Here's how the part is built. I have some questions about the finished solid (model axes, mm). A direction names the side the tool comes from. Round coordinates to 2 decimals unless told otherwise and drop trailing zeros. Order: outer loops, then holes, each group sorted by start corner. A loop starts at its lowest first (then second) coordinate and runs counter-clockwise, first axis right, second up. Notation, with made-up numbers: M 31,80.5 L 58,80.5 A18 cw 58,115.5 Z; hole C 36,-5.75 d4. An arc over 180 degrees is marked long. Write item = value, one per line. Start each with the question number.
Item 1: I want a section at C-C, the plane z = 15.5. List the corners of the cut face in (x, y) for me, plus the area to 3 significant figures.
Item 2: I want a section at D-D, the plane x = 0. List the corners of the cut face in (y, z) for me, plus the area to 3 significant figures.
Item 3: I want a section at A-A, the plane y = 0. State how many separate pieces and enclosed holes the cut face has, plus the area to 3 significant figures.
Item 4: For faces 1 (the face through (0, 5, 48)), 2 (the face through (-19, 0, 29)), 3 (the face through (-17.247, 0.121, 59.479)), which set-ups out of +Z, -Z, +X, -X, +Y, -Y let a thin tool reach every point of the face, with its end or its side?
Item 5: I'm going to push flat-ended pins straight in: P1, Ø6, axis at y = -1, z = 45.5, coming from the -X side; P2, Ø3.5, axis at x = 14.5, y = 0, coming from the +Z side. Where does each tip first touch, or does it pass through?
Item 6: We'd pull the mould along Y, two halves only. Please class faces 4 (the face through (2, -10, 23)), 5 (the face through (-17, -2, 20)), 6 (the face through (20, -2, 48)): pulls with the +Y half, pulls with the -Y half, needs draft (parallel to the pull), parting line crosses it, or undercut.
Item 7: I want a section at B-B, the plane x = -14.5. List the corners of the cut face in (y, z) for me.
Item 8: Please list where these lines run through material, in increasing order: L1, parallel to Z at x = -9.5, y = 1.25; L2, parallel to Z at x = -13, y = -2.75; L3, parallel to Y at x = 5.5, z = 21.5.
```python
from build123d import *

# Parameters (mm, degrees)
F0_W     = 40
F0_H     = 15
F0_R     = 2.5
F0_R_2   = 4.5
F1_DEPTH = 38
F0_H_2   = 5
F2_DEPTH = 61
F3_START = 58
F3_DEPTH = 3
F0_R_3   = 2.75
F4_DEPTH = 20
F5_START = 58
F5_DEPTH = 3


with BuildPart() as f1:
    # F0 (on Top) → F1 (new body)
    with BuildSketch(Plane.XY):
        with Locations((0, -2.5)):
            Rectangle(F0_W, F0_H)
        with Locations((-6.7427190952, -5)):
            Circle(F0_R, mode=Mode.SUBTRACT)
        with Locations((5.2572809048, -5)):
            Circle(F0_R, mode=Mode.SUBTRACT)
        with Locations((-14.5, 0)):
            Circle(F0_R_2, mode=Mode.SUBTRACT)
        with Locations((14.5, 0)):
            Circle(F0_R_2, mode=Mode.SUBTRACT)
    extrude(amount=F1_DEPTH)

    # F0 (on Top) → F2 (join)
    with BuildSketch(Plane.XY):
        Polygon((25, 10), (20, 10), (20, 5), (20, -10), (25, -10), align=None)
        with Locations((0, 7.5)):
            Rectangle(F0_W, F0_H_2)
    extrude(amount=F2_DEPTH)

    # F0 (on Top) → F3 (join)
    with BuildSketch(Plane.XY.offset(F3_START)):
        with Locations((0, -2.5)):
            Rectangle(F0_W, F0_H)
        with Locations((-6.7427190952, -5)):
            Circle(F0_R, mode=Mode.SUBTRACT)
        with Locations((5.2572809048, -5)):
            Circle(F0_R, mode=Mode.SUBTRACT)
        with Locations((-14.5, 0)):
            Circle(F0_R_2, mode=Mode.SUBTRACT)
        with Locations((14.5, 0)):
            Circle(F0_R_2, mode=Mode.SUBTRACT)
    extrude(amount=F3_DEPTH)

    # F0 (on Top) → F4 (join)
    with BuildSketch(Plane.XY):
        with Locations((-14.5, 0)):
            Circle(F0_R_2)
        with Locations((-14.5, 0)):
            Circle(F0_R_3, mode=Mode.SUBTRACT)
        with Locations((14.5, 0)):
            Circle(F0_R_2)
        with Locations((14.5, 0)):
            Circle(F0_R_3, mode=Mode.SUBTRACT)
    extrude(amount=F4_DEPTH)

    # F0 (on Top) → F5 (join)
    with BuildSketch(Plane.XY.offset(F5_START)):
        with Locations((-14.5, 0)):
            Circle(F0_R_2)
        with Locations((-14.5, 0)):
            Circle(F0_R_3, mode=Mode.SUBTRACT)
        with Locations((14.5, 0)):
            Circle(F0_R_2)
        with Locations((14.5, 0)):
            Circle(F0_R_3, mode=Mode.SUBTRACT)
    extrude(amount=F5_DEPTH)


solid = f1.part
```
Filled in:
q1.outline = M -20,-10 L 25,-10 L 25,10 L -20,10 Z; hole C -14.5,0 d5.5; hole C -6.74,-5 d5; hole C 5.26,-5 d5; hole C 14.5,0 d5.5
q1.area = 813 mm^2
q2.outline = M -10,0 L 10,0 L 10,61 L -10,61 L -10,58 L 5,58 L 5,38 L -10,38 Z
q2.area = 920 mm^2
q3.separate_pieces = 5
q3.enclosed_holes = 0
q3.area = 1,370 mm^2
q4.face_1 = -X, -Y
q4.face_2 = none
q4.face_3 = +Z, -Z
q5.P1 = 20
q5.P2 = through
q6.face_4 = pulls with the -Y half
q6.face_5 = undercut
q6.face_6 = needs draft
q7.outline = M -10,0 L -2.75,0 L -2.75,20 L -4.5,20 L -4.5,38 L -10,38 Z; M -10,58 L -2.75,58 L -2.75,61 L -10,61 Z; M 2.75,0 L 10,0 L 10,61 L 2.75,61 L 2.75,58 L 5,58 L 5,38 L 4.5,38 L 4.5,20 L 2.75,20 Z
q8.L1 = 0 to 38, 58 to 61
q8.L2 = 0 to 20, 58 to 61
q8.L3 = -10 to -7.49, -2.51 to 10
